Build history of the part. All positions in model axes, mm. Face numbers are marked on the shaded views. A direction names the side the tool comes from. Give positions to 0.01 mm unless a question says otherwise; leave off trailing zeros. Loops run counter-clockwise (first coordinate to the right, second up) from the corner with the lowest first, then second, coordinate; pieces in that order, holes last. Notation, with made-up numbers: (26, 72) -> (60, 72) arc R21 cw to (60, 80) -> close; hole circle Ø5 at (55.5, -39.75). An arc over 180 degrees is marked (long way). Answer as a JSON object with one key per item and string values. Group by question number.
Autodesk Inventor part; units mm, degrees
ref_plane "YZ Plane" through (0, 0, 0) normal (1, 0, 0) x (0, 1, 0)
ref_plane "XZ Plane" through (0, 0, 0) normal (0, 1, 0) x (-1, 0, 0)
ref_plane "XY Plane" through (0, 0, 0) normal (0, 0, 1) x (1, 0, 0)
sketch "スケッチ1" plane through (0, 0, 0) normal (0, 1, 0) x (-1, 0, 0)
  circle A0 centre (0, 0) radius 7
  circle A1 centre (0, 0) radius 4
  dimension "d0" = 14
  dimension "d1" = 8
extrude "押し出し1" add sketch "スケッチ1" along normal blind 4
sketch "スケッチ2" plane through (0, 4, 0) normal (0, 1, 0) x (1, 0, 0)
  circle A0 centre (0, 0) radius 7
  line L0 (-7, 0) -> (7, 0)
  line L1 (-7, 0.75) -> (7, 0.75)
  line L2 (-7, 0.75) -> (-7, 0)
  line L3 (7, 0.75) -> (7, 0)
  line L4 (-7, -0.75) -> (7, -0.75)
  line L5 (-7, -0.75) -> (-7, 0)
  line L6 (7, -0.75) -> (7, 0)
  point P0 (6.9597, 0.75)
  point P1 (-6.9597, 0.75)
  point P2 (-6.9597, -0.75)
  point P3 (6.9597, -0.75)
  dimension "d4" = 0.75
extrude "押し出し2" cut sketch "スケッチ2" against normal blind 0.3 contours L0 A0 L1 | A0 L4 L0
chamfer "面取り1" distance 0.3 angle 45 6 edges at (0, 4, 4) (0, 4, -4) (0, 4, -7) (0, 4, 7) (7, 0, 0) (4, 0, 0)
properties part number "GSB-081404"
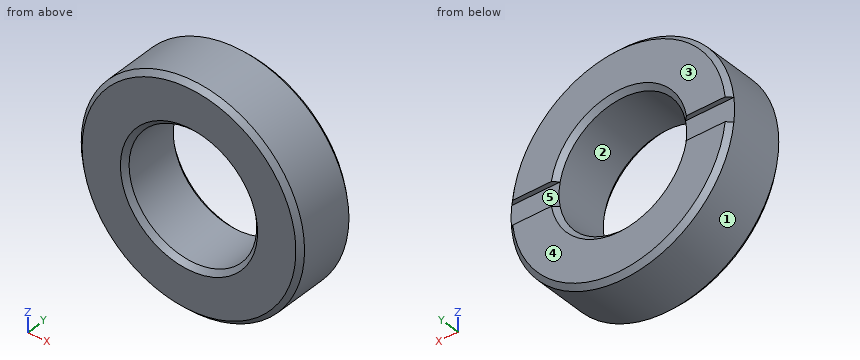
(1) Probe line 1 along X through (y, z) = (2.4, 0.75); line 2 along Z through (x, y) = (0, 3.05); line 3 along Z through (x, y) = (1.5, 2.2). List the from-to ranges inside material, lowest first. Write a range as [from, to].
(2) Saw through at A-A on x = 0. List the corners of the cut face in (y, z), plus the area to 3 significant figures.
(3) Saw through at C-C on y = 2.8. List the corners of the cut face in (x, z).
(4) Pin check, flat tips, straight feed: pin 1 (3 mm diameter, centred on x = -3.5, z = -2, fed in from +Y); pin 2 (7 mm diameter, centred on x = 0, z = 0, fed in from -Y); pin 3 (1.5 mm diameter, centred on y = 3, z = -2, fed in from -X). Stop position of each tip, or through.
(5) 3-axis set-ups, long thin cutter, end or side, ignore diameter. For the marked faces 4 and 5: which of +Z, -Z, +X, -X, +Y, -Y reach the whole face in a straight line?
(6) Saw through at B-B on z = 0. List the corners of the cut face in (x, y), plus the area to 3 significant figures.
(7) Pull direction Z, two halves, no side cores. Call the marked faces 1, 2 and 3: pulls with the +Z half, pulls with the -Z half, needs draft (parallel to the pull), parting line crosses it, or undercut.
Calculated:
{
 "1": {"line 1": "x = [-6.96, -3.93], [3.93, 6.96]", "line 2": "z = [-7, -4], [4, 7]", "line 3": "z = [-6.84, -3.71], [3.71, 6.84]"},
 "2": {"outline": "(0, -6.7) -> (0.3, -7) -> (3.7, -7) -> (4, -6.7) -> (4, -4.3) -> (3.7, -4) -> (0.3, -4) -> (0, -4.3) -> close; (0, 4.3) -> (0.3, 4) -> (3.7, 4) -> (4, 4.3) -> (4, 6.7) -> (3.7, 7) -> (0.3, 7) -> (0, 6.7) -> close", "area": "23.6 mm^2"},
 "3": {"outline": "circle Ø14 at (0, 0); hole circle Ø8 at (0, 0)"},
 "4": {"pin 1": "stops at y = 4", "pin 2": "passes through", "pin 3": "stops at x = -6.89"},
 "5": {"face 4": "+Z, -Z, +X, -X, +Y", "face 5": "+X, -X, +Y"},
 "6": {"outline": "(-7, 0.3) -> (-6.7, 0) -> (-4.3, 0) -> (-4, 0.3) -> (-4, 3.7) -> (-7, 3.7) -> close; (4, 0.3) -> (4.3, 0) -> (6.7, 0) -> (7, 0.3) -> (7, 3.7) -> (4, 3.7) -> close", "area": "22.0 mm^2"},
 "7": {"face 1": "parting line crosses it", "face 2": "undercut", "face 3": "needs draft"}
}
